The model under review builds one solid part; all positions refer to its coordinate system, in mm. Face numbers are marked on the shaded views. A direction names the side the tool comes from. Give positions to 0.01 mm unless a question says otherwise; leave off trailing zeros. Loops run counter-clockwise (first coordinate to the right, second up) from the corner with the lowest first, then second, coordinate; pieces in that order, holes last. Notation, with made-up numbers: (-5, 7) - (6, 7) arc R6 cw to (6, 13) - close; hole circle Ø8 at (-8.75, 78.25). An arc over 180 degrees is marked (long way). Answer as a JSON object with one key per item and string values.
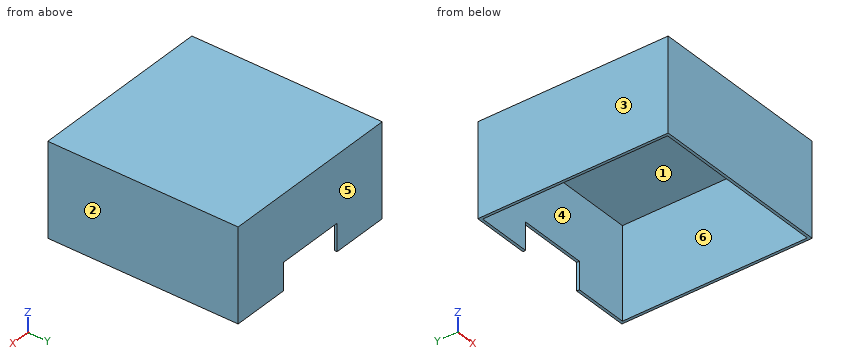
from build123d import *

# Parameters (mm, degrees)
SKETCH_1_W          = 268
SKETCH_1_H          = 136
EXTRUDE_1_DEPTH     = 278
SKETCH_2_W          = 260
SKETCH_2_H          = 270
CUT_EXTRUDE_1_DEPTH = 134
CUT_EXTRUDE_2_REACH = 318.013
SKETCH_3_W          = 100
SKETCH_3_H          = 40


with BuildPart() as part:
    # 草图1 → 凸台-拉伸1 (new body)
    with BuildSketch(Plane(origin=(0, 0, 0), x_dir=(1, 0, 0), z_dir=(0, 1, 0))):
        Rectangle(SKETCH_1_W, SKETCH_1_H)
    extrude(amount=EXTRUDE_1_DEPTH)

    # 草图2 → 切除-拉伸1 (cut)
    with BuildSketch(Plane(origin=(0, 0, -68), x_dir=(-1, 0, 0), z_dir=(0, 0, -1))):
        with Locations((0, 139)):
            Rectangle(SKETCH_2_W, SKETCH_2_H)
    extrude(amount=-CUT_EXTRUDE_1_DEPTH, mode=Mode.SUBTRACT)

    # 草图3 → 切除-拉伸2 (cut, up to next)
    with BuildSketch(Plane(origin=(0, 278, 0), x_dir=(1, 0, 0), z_dir=(0, 1, 0)), mode=Mode.PRIVATE) as cut_extrude_2_sk1:
        with Locations((0, 48)):
            Rectangle(SKETCH_3_W, SKETCH_3_H)
    cut_extrude_2_tool1 = extrude(cut_extrude_2_sk1.sketch, amount=-CUT_EXTRUDE_2_REACH, mode=Mode.PRIVATE) & part.part
    add(cut_extrude_2_tool1.solids().sort_by_distance((0, 278, -48))[0], mode=Mode.SUBTRACT)


solid = part.part
Q1. To check wall thickness, follow probe 1 along X at (y, z) = (62, -49); probe 2 along Y at (x, z) = (-8.5, -12.5); probe 3 along Z at (x, y) = (12.5, 65). State the ranges of each line that lie inside material, in increasing order. Write a range as [from, to].
Results:
{"probe 1": "x = [-134, -130], [130, 134]", "probe 2": "y = [0, 4], [274, 278]", "probe 3": "z = [66, 68]"}
Q2. The part is to be moulded in two halves that separate along X. For the marked faces 3, 4, 5 and 6, say which applies: +X half, -X half, draft (parallel to the pull), parting line (faces both ways), or undercut.
Results:
{"face 3": "-X half", "face 4": "undercut", "face 5": "draft", "face 6": "undercut"}
Q3. Consider section D-D, the plane z = -33. State the section outline as (x, y) points.
Results:
{"outline": "(-134, 0) - (134, 0) - (134, 278) - (50, 278) - (50, 274) - (130, 274) - (130, 4) - (-130, 4) - (-130, 274) - (-50, 274) - (-50, 278) - (-134, 278) - close"}
Q4. Consider section C-C, the plane y = 226.5. State the section outline as (x, z) points.
Results:
{"outline": "(-134, -68) - (-130, -68) - (-130, 66) - (130, 66) - (130, -68) - (134, -68) - (134, 68) - (-134, 68) - close"}
Q5. Consider section A-A, the plane x = -55. State the section outline as (y, z) points, plus the area to 3 significant figures.
Results:
{"outline": "(0, -68) - (4, -68) - (4, 66) - (274, 66) - (274, -68) - (278, -68) - (278, 68) - (0, 68) - close", "area": "1,630 mm^2"}
Q6. Consider section B-B, the plane z = 42. State the section outline as (x, y) points, plus the area to 3 significant figures.
Results:
{"outline": "(-134, 0) - (134, 0) - (134, 278) - (-134, 278) - close; hole (-130, 4) - (130, 4) - (130, 274) - (-130, 274) - close", "area": "4,300 mm^2"}
Q7. For the marked faces 1 and 2, list the 3-axis set-ups (+Z, -Z, +X, -X, +Y, -Y) from which the entire face can be reached by the end or side of a thin tool; tool diameter is ignored.
Results:
{"face 1": "-Z", "face 2": "+Z, -Z, +X, +Y, -Y"}
Q8. Clearance check with flat-ended pins moving along their axes: pin 1 Ø6 at (x, y) = (0, 90.5) entering from -Z; pin 2 Ø1.2 at (x, y) = (-21, 277) entering from -Z. State where each tip first meets the part, or that it passes through.
Results:
{"pin 1": "stops at z = 66", "pin 2": "stops at z = -28"}
